from build123d import *

# Parameters (mm, degrees)
ENL_V_START             = 0.5
ENL_V_MAT_EXTRU_1_DEPTH = 3
CHANFREIN1_SIZE         = 1


with BuildPart() as part:
    # Esquisse1 → Révolution1 (revolve)
    with BuildSketch(Plane.XY, mode=Mode.PRIVATE) as r_volution1_sk:
        with BuildLine():
            Line((0, -12), (0, 2.5))
            ThreePointArc((0, 2.5), (-2.371708245, 2.115124735), (-4.5, 1))
            Line((-4.5, 1), (-4.5, 0))
            Line((-4.5, 0), (-2.5, 0))
            Line((-2.5, 0), (-2.5, -12))
            Line((-2.5, -12), (0, -12))
        make_face()
    revolve(r_volution1_sk.sketch.rotate(Axis((0, 16.1829806, 0), (0, -1, 0)), 270), axis=Axis((0, 16.1829806, 0), (0, -1, 0)))  # turned: the seam where the file's is

    # Esquisse2 → Enlèv. mat.-Extru.1 (cut, through all)
    with BuildSketch(Plane(origin=(0, 0, 0), x_dir=(1, 0, 0), z_dir=(0, 1, 0)).offset(ENL_V_START)):
        Polygon((0, 1.732050808), (-1.5, 0.866025404), (-1.5, -0.866025404), (0, -1.732050808), (1.5, -0.866025404), (1.5, 0.866025404), align=None)
    extrude(amount=ENL_V_MAT_EXTRU_1_DEPTH, mode=Mode.SUBTRACT)

    # Chanfrein1
    chanfrein1_edges = [part.edges().sort_by_distance(p)[0] for p in [
        (0, -12, -2.5),
    ]]
    chamfer(chanfrein1_edges, length=CHANFREIN1_SIZE)


solid = part.part
Verification items for the finished model (mm, model axes). A direction names the side the tool comes from. Coordinates: 2 decimals unless noted, no trailing zeros. Order: outer loops, then holes, each group sorted by start corner. A loop starts at its lowest first (then second) coordinate and runs counter-clockwise, first axis right, second up. Notation, with made-up numbers: (-2.5, -18) -> (12.5, -18) arc R7 ccw to (12.5, -8) -> close; hole circle Ø8 at (40, 9.25). An arc over 180 degrees is marked (long way). Use CSV: the item, a comma, the result in double quotes. Start each with the question number.
Q1. Draft check along Z on faces 1 (the cylindrical face through (2.44, -5.58, -0.54)), 2 (the flat face through (-1.5, 1, 0)), 3 (the flat face through (-0.739, 1.411, -1.305)), 4 (the flat face through (0, -12, 0)). Enter one of: +Z half, -Z half, draft (parallel to the pull), parting line (faces both ways), or undercut.
Q2. Thickness scan on line 1 along Y through (x, z) = (1, 0.25); line 2 along X through (y, z) = (-5.5, 2); line 3 along Z through (x, y) = (0.5, -5.75). Record the ranges inside material, lowest first.
Q3. Section check D-D, the plane z = 2.75. Record the cut outline in (x, y), and give its area (3 significant figures).
Q4. Section check B-B, the plane y = -1. Record the cut outline in (x, z), and give its area (3 significant figures).
Q5. Tool access check on faces 5 (the flat face through (-0.76, 1.411, 1.293)), 6 (the cylindrical face through (-1.352, 0.493, 4.292)), 7 (the flat face through (2, 0, 2)). Record the directions out of +Z, -Z, +X, -X, +Y, -Y that give a thin tool (end or side, any length) a straight path to the whole face; none if there is none.
Q6. Section check C-C, the plane x = -3.5. Record the cut outline in (y, z), and give its area (3 significant figures).
Q7. Section check A-A, the plane z = 0. Record the cut outline in (x, y).
Q8. Depth check by flat-ended pin: P1, Ø1, axis at x = 2.5, y = -1.5, coming from the -Z side; P2, Ø4, axis at y = -9, z = 1, coming from the +X side; P3, Ø0.9, axis at x = 0, z = -0.5, coming from the +Y side. Enter the tip coordinate at first touch or a pass-through.
Returned:
1,face 1,"parting line"
1,face 2,"undercut"
1,face 3,"undercut"
1,face 4,"draft"
2,line 1,"y = -12 to 0.5"
2,line 2,"x = -1.5 to 1.5"
2,line 3,"z = -2.45 to 2.45"
3,outline,"(-3.56, 0) -> (3.56, 0) -> (3.56, 1) arc R6.98 ccw to (-3.56, 1) -> close"
3,area,"11.8 mm^2"
4,outline,"circle Ø5 at (0, 0)"
4,area,"19.6 mm^2"
5,face 5,"+Y"
5,face 6,"+Y, -Y"
5,face 7,"-Y"
6,outline,"(0, -2.83) -> (1, -2.83) arc R6.63 ccw to (1, 2.83) -> (0, 2.83) -> close"
6,area,"8.07 mm^2"
7,outline,"(-4.5, 0) -> (-2.5, 0) -> (-2.5, -11) -> (-1.5, -12) -> (1.5, -12) -> (2.5, -11) -> (2.5, 0) -> (4.5, 0) -> (4.5, 1) arc R7.5 ccw to (1.5, 2.35) -> (1.5, 0.5) -> (-1.5, 0.5) -> (-1.5, 2.35) arc R7.5 ccw to (-4.5, 1) -> close"
8,P1,"stops at z = -1.5"
8,P2,"stops at x = 2.5"
8,P3,"stops at y = 0.5"
